Check sheet for the modelled part. Datum: model origin and axes. Units: mm. Round coordinates to 2 decimals unless told otherwise and drop trailing zeros. Order: outer loops, then holes, each group sorted by start corner. A loop starts at its lowest first (then second) coordinate and runs counter-clockwise, first axis right, second up. Notation, with made-up numbers: (85, 71) -> (120, 71) arc R12 ccw to (120, 82) -> close; hole circle Ø6 at (-18.75, 61). An arc over 180 degrees is marked (long way). Answer in a Markdown table with one row per item.
```python
from build123d import *

# Parameters (mm, degrees)
EXTRUDE_1_DEPTH        = 210
SKETCH_2_R             = 3
CUT_EXTRUDE_1_DEPTH    = 4.5
SKETCH_4_R             = 1.75
CUT_EXTRUDE_2_DEPTH    = 211.205851488
PATTERN_LINEAR_1_COUNT = 15
PATTERN_LINEAR_1_PITCH = 40


with BuildPart() as part:
    # 草图1 → 凸台-拉伸1 (new, symmetric)
    with BuildSketch(Plane(origin=(0, 0, 0), x_dir=(0, 0, -1), z_dir=(1, 0, 0))):
        with BuildLine():
            Line((-7.5, 5), (-7.5, 0.4))
            Line((-7.5, 0.4), (-7.1, 0))
            Line((-7.1, 0), (0.7, 0))
            ThreePointArc((0.7, 0), (1, 0.3), (1.3, 0))
            Line((1.3, 0), (7.1, 0))
            Line((7.1, 0), (7.5, 0.4))
            Line((7.5, 0.4), (7.5, 5))
            ThreePointArc((7.5, 5), (6.439339828, 5.439339828), (6, 6.5))
            ThreePointArc((6, 6.5), (6.439339828, 7.560660172), (7.5, 8))
            Line((7.5, 8), (7.5, 9.6))
            Line((7.5, 9.6), (7.1, 10))
            Line((7.1, 10), (-7.1, 10))
            Line((-7.1, 10), (-7.5, 9.6))
            Line((-7.5, 9.6), (-7.5, 8))
            ThreePointArc((-7.5, 8), (-6.439339823, 7.560660166), (-6, 6.499999984))
            ThreePointArc((-6, 6.499999984), (-6.439339834, 5.439339823), (-7.5, 5))
        make_face()
    extrude(amount=EXTRUDE_1_DEPTH, both=True)

    # 草图2 → 切除-拉伸1 (cut)
    with BuildSketch(Plane(origin=(0, 10, 0), x_dir=(1, 0, 0), z_dir=(0, 1, 0))):
        with Locations(Location((-180, 0, 0), (0, 0, 270))):
            Circle(SKETCH_2_R)
    cut_extrude_1 = extrude(amount=-CUT_EXTRUDE_1_DEPTH, mode=Mode.SUBTRACT)

    # 草图4 → 切除-拉伸2 (cut, through all)
    with BuildSketch(Plane(origin=(0, 5.5, 0), x_dir=(1, 0, 0), z_dir=(0, 1, 0))):
        with Locations(Location((-180, 0, 0), (0, 0, 270))):
            Circle(SKETCH_4_R)
    cut_extrude_2 = extrude(amount=-CUT_EXTRUDE_2_DEPTH, mode=Mode.SUBTRACT)

    # 阵列(线性)1: 切除-拉伸1, 切除-拉伸2 ×15
    with Locations(*[(i * PATTERN_LINEAR_1_PITCH, 0, 0) for i in range(1, PATTERN_LINEAR_1_COUNT)]):
        add(cut_extrude_1, mode=Mode.SUBTRACT)
        add(cut_extrude_2, mode=Mode.SUBTRACT)


solid = part.part
```
(1) Scan lines: probe 1 along Z at (x, y) = (180, 2.45); probe 2 along Z at (x, y) = (100, 8.5); probe 3 along Y at (x, z) = (2, 6.5). Record each from-to range of solid material in increasing order. Write a range as from..to.
Solutions:
| item | result |
|---|---|
| probe 1 | -7.5..-1.75, 1.75..7.5 |
| probe 2 | -7.5..-3, 3..7.5 |
| probe 3 | 0..5.38, 7.62..10 |
(2) Section check B-B on x = 109. Record the boundary of the cut face in (y, z).
Solutions:
| item | result |
|---|---|
| outline | (0, -7.1) -> (0.4, -7.5) -> (5, -7.5) arc R1.5 cw to (8, -7.5) -> (9.6, -7.5) -> (10, -7.1) -> (10, 7.1) -> (9.6, 7.5) -> (8, 7.5) arc R1.5 cw to (5, 7.5) -> (0.4, 7.5) -> (0, 7.1) -> (0, -0.7) arc R0.3 cw to (0, -1.3) -> close |
(3) Depth check by flat-ended pin: pin 1 Ø3 at (x, z) = (-140, 0) entering from -Y; pin 2 Ø3 at (x, z) = (139, 0) entering from +Y. Enter the tip coordinate at first touch or a pass-through.
Solutions:
| item | result |
|---|---|
| pin 1 | through |
| pin 2 | y = 5.5 |
(4) Section check A-A on y = 3. Give the number of separate pieces and of enclosed holes in the cut face, plus the area to 3 significant figures.
Solutions:
| item | result |
|---|---|
| separate pieces | 1 |
| enclosed holes | 10 |
| area | 6,200 mm^2 |
